from build123d import *

# Parameters (mm, degrees)
F0_R     = 4
F1_DEPTH = 10
F2_R     = 6
F3_DEPTH = 2
F4_R     = 1


with BuildPart() as f1:
    # F0 (on Front) → F1 (new body)
    with BuildSketch(Plane.XZ):
        Circle(F0_R)
    extrude(amount=F1_DEPTH)

    # F2 (on face) → F3 (join)
    with BuildSketch(Plane.XZ.offset(10)):
        Circle(F2_R)
    extrude(amount=F3_DEPTH)

    # F4
    f4_edges = [f1.edges().sort_by_distance(p)[0] for p in [
        (-4, 0, 0),
        (-6, -12, 0),
    ]]
    fillet(f4_edges, radius=F4_R)


solid = f1.part
Part model, mm, in its own coordinate system. Coordinates: 2 decimals unless noted, no trailing zeros. Loops run counter-clockwise (first coordinate to the right, second up) from the corner with the lowest first, then second, coordinate; pieces in that order, holes last. Notation, with made-up numbers: (69.5, -35.5) -> (79.5, -35.5) arc R13 ccw to (79.5, -28.5) -> close; hole circle Ø7 at (37, 61). An arc over 180 degrees is marked (long way). Use a Markdown table: item, result. Add a question column.
Item 1: Band-saw the part on A-A on z = 0. Write the cut outline in (x, y).
Item 2: Band-saw the part on B-B on x = 0. Write the cut outline in (y, z), plus the area to 3 significant figures.
Item 3: Flat gauge pins, fed straight in: P1, Ø1.5, axis at y = -7.5, z = 0.5, coming from the +X side; P2, Ø2, axis at y = -9.5, z = -2.5, coming from the +X side; P3, Ø1.5, axis at x = 4, z = 3, coming from the +Y side. Where does each tip first touch, or does it go through?
Item 4: Pull direction Y, two halves, no side cores. Call faces 1 (the flat face through (0, -12, 0)), 2 (the cylindrical face through (-0.867, -5.437, -3.905)), 3 (the flat face through (-1.42, -10, -3.92)): +Y half, -Y half, draft (parallel to the pull), parting line (faces both ways), or undercut.
Item 5: Probe probe 1 along Y at (x, z) = (-1.25, -4.5); probe 2 along Z at (x, y) = (3.5, -9.5). List the from-to ranges inside material, lowest first.
Item 6: Band-saw the part on C-C on y = -5.25. Write the cut outline in (x, z), plus the area to 3 significant figures.
Geometry says:
| question | item | result |
|---|---|---|
| 1 | outline | (-6, -11) arc R1 ccw to (-5, -12) -> (5, -12) arc R1 ccw to (6, -11) -> (6, -10) -> (4, -10) -> (4, -1) arc R1 ccw to (3, 0) -> (-3, 0) arc R1 ccw to (-4, -1) -> (-4, -10) -> (-6, -10) -> close |
| 2 | outline | (-12, -5) arc R1 ccw to (-11, -6) -> (-10, -6) -> (-10, -4) -> (-1, -4) arc R1 ccw to (0, -3) -> (0, 3) arc R1 ccw to (-1, 4) -> (-10, 4) -> (-10, 6) -> (-11, 6) arc R1 ccw to (-12, 5) -> close |
| 2 | area | 103 mm² |
| 3 | P1 | x = 4 |
| 3 | P2 | x = 5.77 |
| 3 | P3 | y = -10 |
| 4 | face 1 | -Y half |
| 4 | face 2 | draft |
| 4 | face 3 | +Y half |
| 5 | probe 1 | -12 to -10 |
| 5 | probe 2 | -1.94 to 1.94 |
| 6 | outline | circle Ø8 at (0, 0) |
| 6 | area | 50.3 mm² |
